Here's how the part is built. I have some questions about the finished solid (model axes, mm). Face numbers are marked on the shaded views. Coordinates: 2 decimals unless noted, no trailing zeros. Write each loop counter-clockwise with the first axis right and the second up, starting at its lowest first coordinate (ties: lowest second). Pieces come first, ordered by that corner, then holes. Notation, with made-up numbers: (52, -38.5) -> (80, -38.5) arc R21 cw to (80, -15.5) -> close; hole circle Ø10 at (44, 65.5). An arc over 180 degrees is marked (long way). Put each result on its own line as item: value. Start each with the question number.
Item 1: I need wall thicknesses on line 1 (Y direction, x = 20.5, z = 7.75); line 2 (Z direction, x = 6, y = 8). Which ranges of each line are inside material? Lowest first, please. Write a range as [from, to].
Item 2: I want a section at B-B, the plane x = 11.29. List the corners of the cut face in (y, z) for me.
Item 3: I want a section at A-A, the plane y = 9.5. State how many separate pieces and enclosed holes the cut face has, then the cut area to 3 significant figures.
Item 4: If we mould it in two halves opening along Z, with no side actions, what happens to the marked faces 1, 2, 3 and 4? For each: released by +Z, released by -Z, zero draft, split by the parting line, or undercut.
Item 5: I want a section at C-C, the plane z = 3.25. List the corners of the cut face in (x, y) for me, then the cut area to 3 significant figures.
Item 6: For pin 1 (8 mm diameter, centred on x = 9, z = 9, fed in from +Y), with a flat end and sliding along its axis, tell me the tip position at first contact or that it passes through.
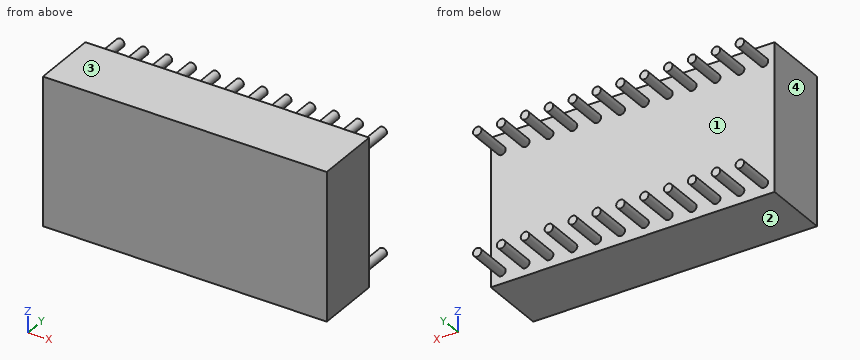
from build123d import *

# Parameters (mm, degrees)
SKETCH1_W           = 30.2
SKETCH1_H           = 15.7
BOSS_EXTRUDE1_DEPTH = 7
SKETCH2_R           = 0.45
BOSS_EXTRUDE2_DEPTH = 4


with BuildPart() as part:
    # Sketch1 → Boss-Extrude1 (new body)
    with BuildSketch(Plane(origin=(0, 0, 0), x_dir=(1, 0, 0), z_dir=(0, 1, 0))):
        with Locations((15.1, -7.85)):
            Rectangle(SKETCH1_W, SKETCH1_H)
    extrude(amount=BOSS_EXTRUDE1_DEPTH)

    # Sketch2 → Boss-Extrude2 (add)
    with BuildSketch(Plane(origin=(0, 7, 0), x_dir=(1, 0, 0), z_dir=(0, 1, 0))):
        with Locations((1.13, -1.25)):
            Circle(SKETCH2_R)
        with Locations((3.67, -1.25)):
            Circle(SKETCH2_R)
        with Locations((6.21, -1.25)):
            Circle(SKETCH2_R)
        with Locations((8.75, -1.25)):
            Circle(SKETCH2_R)
        with Locations((11.29, -1.25)):
            Circle(SKETCH2_R)
        with Locations((13.83, -1.25)):
            Circle(SKETCH2_R)
        with Locations((16.37, -1.25)):
            Circle(SKETCH2_R)
        with Locations((18.91, -1.25)):
            Circle(SKETCH2_R)
        with Locations((21.45, -1.25)):
            Circle(SKETCH2_R)
        with Locations((23.99, -1.25)):
            Circle(SKETCH2_R)
        with Locations((26.53, -1.25)):
            Circle(SKETCH2_R)
        with Locations((29.07, -1.25)):
            Circle(SKETCH2_R)
        with Locations((29.07, -13.95)):
            Circle(SKETCH2_R)
        with Locations((26.53, -13.95)):
            Circle(SKETCH2_R)
        with Locations((23.99, -13.95)):
            Circle(SKETCH2_R)
        with Locations((21.45, -13.95)):
            Circle(SKETCH2_R)
        with Locations((18.91, -13.95)):
            Circle(SKETCH2_R)
        with Locations((16.37, -13.95)):
            Circle(SKETCH2_R)
        with Locations((13.83, -13.95)):
            Circle(SKETCH2_R)
        with Locations((11.29, -13.95)):
            Circle(SKETCH2_R)
        with Locations((8.75, -13.95)):
            Circle(SKETCH2_R)
        with Locations((6.21, -13.95)):
            Circle(SKETCH2_R)
        with Locations((3.67, -13.95)):
            Circle(SKETCH2_R)
        with Locations((1.13, -13.95)):
            Circle(SKETCH2_R)
    extrude(amount=BOSS_EXTRUDE2_DEPTH)


solid = part.part
Calculated:
1. line 1: y = [0, 7]
1. line 2: z = [0.85, 1.65], [13.55, 14.35]
2. outline: (0, 0) -> (7, 0) -> (7, 0.8) -> (11, 0.8) -> (11, 1.7) -> (7, 1.7) -> (7, 13.5) -> (11, 13.5) -> (11, 14.4) -> (7, 14.4) -> (7, 15.7) -> (0, 15.7) -> close
3. separate pieces: 24
3. enclosed holes: 0
3. area: 15.3 mm2
4. face 1: undercut
4. face 2: released by -Z
4. face 3: released by +Z
4. face 4: zero draft
5. outline: (0, 0) -> (30.2, 0) -> (30.2, 7) -> (0, 7) -> close
5. area: 211 mm2
6. pin 1: stops at y = 7
